Input: part model. Units: mm. Frame: model coordinates. A direction names the side the tool comes from. Give positions to 0.01 mm unless a question says otherwise; leave off trailing zeros. Loops run counter-clockwise (first coordinate to the right, second up) from the corner with the lowest first, then second, coordinate; pieces in that order, holes last. Notation, with made-up numbers: (67.25, -36.75) - (103.25, -36.75) arc R24 ccw to (103.25, -1.75) - close; hole circle Ø8 at (-18, 78.5). An arc over 180 degrees is marked (long way). Answer as a JSON object with one key per item and string values.
from build123d import *

# Parameters (mm, degrees)
SKETCH1_R                = 5
BOSS_EXTRUDE1_DEPTH      = 5
BOSS_EXTRUDE1_DEPTH_BACK = 45
SKETCH2_W                = 5
SKETCH2_H                = 10
CUT_EXTRUDE1_DEPTH       = 6
CUT_EXTRUDE1_DEPTH_BACK  = 6


with BuildPart() as part:
    # Sketch1 → Boss-Extrude1 (new body, two sides)
    with BuildSketch(Plane(origin=(0, 0, 0), x_dir=(1, 0, 0), z_dir=(0, 1, 0))) as boss_extrude1_sk:
        Circle(SKETCH1_R)
    extrude(amount=BOSS_EXTRUDE1_DEPTH)
    extrude(boss_extrude1_sk.sketch, amount=-BOSS_EXTRUDE1_DEPTH_BACK)

    # Sketch2 → Cut-Extrude1 (cut, two sides)
    with BuildSketch(Plane(origin=(0, 0, 0), x_dir=(0, 0, -1), z_dir=(1, 0, 0))) as cut_extrude1_sk:
        Rectangle(SKETCH2_W, SKETCH2_H)
    extrude(amount=CUT_EXTRUDE1_DEPTH, mode=Mode.SUBTRACT)
    extrude(cut_extrude1_sk.sketch, amount=-CUT_EXTRUDE1_DEPTH_BACK, mode=Mode.SUBTRACT)


solid = part.part
Item 1: Access query for faces 5 (the face through (0, 0, -2.5)), 6 (the face through (0, 5, 3)). Directions: +Z, -Z, +X, -X, +Y, -Y. A direction counts if a zero-diameter tool reaches every point of the face in a straight line with its end or side. Return the directions, or none.
Geometry check:
{"face 5": "+X, -X, +Y", "face 6": "+Z, -Z, +X, -X, +Y"}
Item 2: Contact query for flat-ended pins moving along their axis: P1, Ø2.5, axis at x = 2, y = 2, coming from the +Z side; P2, Ø2, axis at x = -2.5, y = -4.5, coming from the -Z side; P3, Ø2.5, axis at x = -1.5, z = -0.5, coming from the +Y side. Output: stop coordinate, or through.
Geometry check:
{"P1": "stops at z = 4.94", "P2": "stops at z = -4.77", "P3": "stops at y = -5"}
Item 3: Cut plane B-B (y = -8.5). Return loops of the section in (x, z), then the cut area to 3 significant figures.
Geometry check:
{"outline": "circle Ø10 at (0, 0)", "area": "78.5 mm2"}
Item 4: Material intervals for line 1 (Y direction, x = -4.25, z = -2.25); line 2 (Z direction, x = -0.25, y = -40); line 3 (Z direction, x = -2.75, y = -2), sorted ascending. Write a range as [from, to].
Geometry check:
{"line 1": "y = [-45, -5]", "line 2": "z = [-4.99, 4.99]", "line 3": "z = [-4.18, -2.5], [2.5, 4.18]"}
Item 5: Cut plane D-D (z = -3). Return loops of the section in (x, y).
Geometry check:
{"outline": "(-4, -45) - (4, -45) - (4, 5) - (-4, 5) - close"}
Item 6: Cut plane A-A (x = 0). Return loops of the section in (y, z), then the cut area to 3 significant figures.
Geometry check:
{"outline": "(-45, -5) - (5, -5) - (5, -2.5) - (-5, -2.5) - (-5, 2.5) - (5, 2.5) - (5, 5) - (-45, 5) - close", "area": "450 mm2"}
Item 7: Cut plane C-C (x = -2.5). Return loops of the section in (y, z).
Geometry check:
{"outline": "(-45, -4.33) - (5, -4.33) - (5, -2.5) - (-5, -2.5) - (-5, 2.5) - (5, 2.5) - (5, 4.33) - (-45, 4.33) - close"}
Item 8: Mould query, pull axis Z, two halves, no side actions, for faces 1 (the face through (0, 0, 2.5)), 2 (the face through (-5, -20, 0)), 3 (the face through (0, -45, 0)), 4 (the face through (0, -5, 0)). Classes: released by +Z, released by -Z, zero draft, split by the parting line, or undercut.
Geometry check:
{"face 1": "undercut", "face 2": "split by the parting line", "face 3": "zero draft", "face 4": "undercut"}
